Autodesk Inventor part; units mm, degrees
ref_plane "YZ Plane" through (0, 0, 0) normal (1, 0, 0) x (0, 1, 0)
ref_plane "XZ Plane" through (0, 0, 0) normal (0, 1, 0) x (-1, 0, 0)
ref_plane "XY Plane" through (0, 0, 0) normal (0, 0, 1) x (1, 0, 0)
sketch "Sketch1" plane through (0, 0, 0) normal (0, 1, 0) x (-1, 0, 0)
  circle A0 centre (0, 0) radius 1.115 construction
  arc A1 (-0.35, 1.3297) -> (-0.35, -1.3297) centre (0, 0) ccw
  circle A2 centre (0, 0) radius 4.5
  line L0 (0.35, 2) -> (-0.35, 2)
  line L1 (-0.35, 2) -> (-0.35, -2)
  line L2 (-0.35, -2) -> (0.35, -2)
  line L3 (0.35, -2) -> (0.35, 2)
  arc A3 (0.35, 1.3297) -> (-0.35, 1.3297) centre (0, 0) ccw
  arc A4 (0.35, -1.3297) -> (0.35, 1.3297) centre (0, 0) ccw
  arc A5 (-0.35, -1.3297) -> (0.35, -1.3297) centre (0, 0) ccw
  point P0 (0, 2)
  point P1 (0.35, 0)
  dimension "d1" = 2.23
  dimension "d3" = 9
  dimension "d18" = 0.26
  dimension "d19" = 0.7
  dimension "d20" = 4
extrude "Extrusion1" add sketch "Sketch1" along normal blind 3.5
sketch "Sketch4" plane through (0, 0, 0) normal (0, 0, 1) x (1, 0, 0)
  line L0 (-4.2, 17.5) -> (-4.2, 10.5)
  arc A0 (-4.2, 10.5) -> (4.2, 10.5) centre (0, 10.5) ccw
  line L1 (4.2, 10.5) -> (4.2, 17.5)
  line L2 (-3, 17.5) -> (-3, 14.8028)
  arc A1 (-3, 10.5) -> (3, 10.5) centre (0, 10.5) ccw
  line L3 (3, 10.5) -> (3, 11.1972)
  line L4 (-4.2, 17.5) -> (-3, 17.5)
  line L5 (3, 17.5) -> (4.2, 17.5)
  line L6 (-0.35, 0) -> (0.35, 0)
  line L7 (4.5, 3.5) -> (-4.5, 3.5)
  circle A2 centre (0, 13) radius 3.5
  line L8 (-3, 14.8028) -> (-3, 11.1972)
  line L9 (-3, 11.1972) -> (-3, 10.5)
  line L10 (3, 11.1972) -> (3, 14.8028)
  line L11 (3, 14.8028) -> (3, 17.5)
  point P0 (0, 0)
  point P1 (0, 0)
  dimension "d21" = 3
  dimension "d23" = 1.2
  dimension "d24" = 7
  dimension "d25" = 7
  dimension "d26" = 7
  dimension "d27" = 2.5
extrude "Extrusion5" add sketch "Sketch4" along normal mid plane 9 contours L4 L2 A2 L9 A1 L3 L11 L5 L1 A0 L0
sketch "Sketch8" plane through (0, 3.5, 0) normal (0, 1, 0) x (1, 0, 0)
  circle A0 centre (0, 0) radius 4
  dimension "d33" = 8
extrude "Extrusion6" add sketch "Sketch8" along normal up to next
sketch "Sketch2" plane through (0, 3.5, 0) normal (0, 1, 0) x (1, 0, 0)
  circle A0 centre (0, 0) radius 1.375
  circle A1 centre (0, 0) radius 3.375
  dimension "d6" = 2
  dimension "d9" = 7.3
  dimension "d10" = 2
properties part number "Laser Mount Mk2"
Verification items for the finished model (mm, model axes). A direction names the side the tool comes from. Coordinates: 2 decimals unless noted, no trailing zeros. Write each loop counter-clockwise with the first axis right and the second up, starting at its lowest first coordinate (ties: lowest second). Pieces come first, ordered by that corner, then holes. Notation, with made-up numbers: M 15,73 L 46,73 A19 cw 46,110 Z; hole C 42.25,64.25 d6. An arc over 180 degrees is marked long. Answer as a JSON object with one key per item and string values. Group by question number.
(1) Release check for a two-part mould opening along Y. For faces 1 (the face through (3, 3.5, -3)), 2 (the face through (-3, 16, 0)), 3 (the face through (0, 3.5, 0)) record: +Y half, -Y half, draft (parallel to the pull), parting line (faces both ways), or undercut.
(2) Tool access check on faces 4 (the face through (-4.2, 14, 0)), 5 (the face through (1.375, 1.726, -0.025)), 6 (the face through (4.2, 14, 0)). Record the directions out of +Z, -Z, +X, -X, +Y, -Y that give a thin tool (end or side, any length) a straight path to the whole face; none if there is none.
(3) Cross-section at D-D, the plane x = 3.25. Record the cut outline in (y, z).
(4) Material ranges on line 1 (X direction, y = 15.75, z = -1); line 2 (Z direction, x = -1, y = 2); line 3 (X direction, y = 12.75, z = 2.5), recorded low to high.
(5) Cross-section at C-C, the plane z = 0. Record the cut outline in (x, y) (3 decimals).
(6) Gauge pin test, flat ends, axial feed: pin 1 (3 mm diameter, centred on y = 14.5, z = 1.5, fed in from +X); pin 2 (0.6 mm diameter, centred on y = 11, z = -0.5, fed in from -X); pin 3 (1.5 mm diameter, centred on y = 6.5, z = -1, fed in from -X). Record the tip position at first contact, or that the pin passes through.
(7) Cross-section at A-A, the plane y = 10.75. Record the cut outline in (x, z), and give its area (3 significant figures).
(8) Cross-section at B-B, the plane x = 0. Record the cut outline in (y, z), and give its area (3 significant figures).
Reply:
{
 "1": {"face 1": "undercut", "face 2": "draft", "face 3": "-Y half"},
 "2": {"face 4": "+Z, -Z, -X, +Y", "face 5": "-Y", "face 6": "+Z, -Z, +X, +Y"},
 "3": {"outline": "M 0,-3.11 L 3.5,-3.11 L 3.5,-2.33 L 7.84,-2.33 L 7.84,-4.5 L 11.7,-4.5 L 11.7,4.5 L 7.84,4.5 L 7.84,2.33 L 3.5,2.33 L 3.5,3.11 L 0,3.11 Z; M 14.3,-4.5 L 17.5,-4.5 L 17.5,4.5 L 14.3,4.5 Z"},
 "4": {"line 1": "-4.2 to -3, 3 to 4.2", "line 2": "-4.39 to -0.94, 0.94 to 4.39", "line 3": "-4.2 to -3.49, 3.49 to 4.2"},
 "5": {"outline": "M -4.5,0 L -1.375,0 L -1.375,3.5 L 1.375,3.5 L 1.375,0 L 4.5,0 L 4.5,3.5 L 4,3.5 L 4,9.219 A4.2 ccw 4.2,10.5 L 4.2,17.5 L 3,17.5 L 3,14.803 A3.5 cw 3,11.197 L 3,10.5 A3 cw -3,10.5 L -3,11.197 A3.5 cw -3,14.803 L -3,17.5 L -4.2,17.5 L -4.2,10.5 A4.2 ccw -4,9.219 L -4,3.5 L -4.5,3.5 Z"},
 "6": {"pin 1": "x = 4.2", "pin 2": "x = -4.2", "pin 3": "x = -3.99"},
 "7": {"outline": "M -4.2,-4.5 L -3,-4.5 L -3,4.5 L -4.2,4.5 Z; M 3,-4.5 L 4.2,-4.5 L 4.2,4.5 L 3,4.5 Z", "area": "21.6 mm²"},
 "8": {"outline": "M 0,-4.5 L 3.5,-4.5 L 3.5,-4 L 6.3,-4 L 6.3,-4.5 L 7.5,-4.5 L 7.5,4.5 L 6.3,4.5 L 6.3,4 L 3.5,4 L 3.5,4.5 L 0,4.5 L 0,2 L 3.5,2 L 3.5,-2 L 0,-2 Z", "area": "50.7 mm²"}
}
